Check sheet for the modelled part. Datum: model origin and axes. Units: mm. A direction names the side the tool comes from. Coordinates: 2 decimals unless noted, no trailing zeros. Write each loop counter-clockwise with the first axis right and the second up, starting at its lowest first coordinate (ties: lowest second). Pieces come first, ordered by that corner, then holes. Notation, with made-up numbers: (38.5, 76.25) -> (62.5, 76.25) arc R16 cw to (62.5, 97.25) -> close; hole circle Ø9 at (-5, 29.25). An arc over 180 degrees is marked (long way). One line per item, written item: value. Start each with the question number.
1) Gauge pin test, flat ends, axial feed: P1, Ø8, axis at x = 54.5, y = 98, coming from the +Z side; P2, Ø2, axis at x = 46, y = 105, coming from the -Z side; P3, Ø2, axis at x = -52, y = 67, coming from the -Z side. Record the tip position at first contact, or that the pin passes through.
2) Set-up check for faces 4 (the cylindrical face through (-11.573, 150.266, -88.143)), 5 (the flat face through (-88.9, 151, 12)): record each of +Z, -Z, +X, -X, +Y, -Y from which the full face is reachable in a straight line by a thin tool's end or side.
3) Sectioned sample at D-D on y = 273. Enter the section's corners in (x, z) (3 decimals), plus the area to 3 significant figures.
4) Sectioned sample at B-B on z = 17. Enter the section's corners in (x, y).
5) Sectioned sample at A-A on x = 0. Enter the section's corners in (y, z) (3 decimals), plus the area to 3 significant figures.
6) Draft check along Y on faces 1 (the flat face through (-75.5, 0, -48.2)), 2 (the flat face through (88.9, 151, 12)), 3 (the flat face through (-75.5, 304.8, -48.2)). Enter one of: +Y half, -Y half, draft (parallel to the pull), parting line (faces both ways), or undercut.
7) Sectioned sample at C-C on z = 61.5. Enter the section's corners in (x, y), plus the area to 3 significant figures.
8) Scan lines: line 1 along Y through (x, z) = (81, 40.5); line 2 along X through (y, z) = (109, 0) (3 decimals); line 3 along Z through (x, y) = (-3.5, 85). Record each from-to range of solid material in increasing order. Write a range as [from, to].
```python
from build123d import *

# Parameters (mm, degrees)
SKETCH1_R           = 92.075
SKETCH1_R_2         = 88.9
BOSS_EXTRUDE1_DEPTH = 304.8
SKETCH2_W           = 177.8
SKETCH2_H           = 203.2
CUT_EXTRUDE1_DEPTH  = 93.075


with BuildPart() as part:
    # Sketch1 → Boss-Extrude1 (new body)
    with BuildSketch(Plane(origin=(0, 0, 0), x_dir=(1, 0, 0), z_dir=(0, 1, 0))):
        Circle(SKETCH1_R)
        Circle(SKETCH1_R_2, mode=Mode.SUBTRACT)
    extrude(amount=BOSS_EXTRUDE1_DEPTH)

    # Sketch2 → Cut-Extrude1 (cut, through all)
    with BuildSketch(Plane.XY):
        with Locations((0, 152.4)):
            Rectangle(SKETCH2_W, SKETCH2_H)
    extrude(amount=CUT_EXTRUDE1_DEPTH, mode=Mode.SUBTRACT)


solid = part.part
```
Answers:
1. P1: stops at z = -66.94
1. P2: stops at z = -80.33
1. P3: stops at z = -76.66
2. face 4: +Y, -Y
2. face 5: +Z
3. outline: circle Ø184.15 at (0, 0); hole circle Ø177.8 at (0, 0)
3. area: 1,810 mm2
4. outline: (-90.49, 0) -> (-87.26, 0) -> (-87.26, 50.8) -> (-88.9, 50.8) -> (-88.9, 254) -> (-87.26, 254) -> (-87.26, 304.8) -> (-90.49, 304.8) -> close; (87.26, 0) -> (90.49, 0) -> (90.49, 304.8) -> (87.26, 304.8) -> (87.26, 254) -> (88.9, 254) -> (88.9, 50.8) -> (87.26, 50.8) -> close
5. outline: (0, -92.075) -> (304.8, -92.075) -> (304.8, -88.9) -> (0, -88.9) -> close; (0, 88.9) -> (50.8, 88.9) -> (50.8, 92.075) -> (0, 92.075) -> close; (254, 88.9) -> (304.8, 88.9) -> (304.8, 92.075) -> (254, 92.075) -> close
5. area: 1,290 mm2
6. face 1: -Y half
6. face 2: undercut
6. face 3: +Y half
7. outline: (-68.52, 0) -> (-64.19, 0) -> (-64.19, 50.8) -> (-68.52, 50.8) -> close; (-68.52, 254) -> (-64.19, 254) -> (-64.19, 304.8) -> (-68.52, 304.8) -> close; (64.19, 0) -> (68.52, 0) -> (68.52, 50.8) -> (64.19, 50.8) -> close; (64.19, 254) -> (68.52, 254) -> (68.52, 304.8) -> (64.19, 304.8) -> close
7. area: 880 mm2
8. line 1: y = [0, 50.8], [254, 304.8]
8. line 2: x = [-92.075, -88.9], [88.9, 92.075]
8. line 3: z = [-92.01, -88.83]
